from build123d import *

# Parameters (mm, degrees)
SKETCH1_W           = 100
SKETCH1_H           = 60
BOSS_EXTRUDE1_DEPTH = 5
CUT_EXTRUDE2_START  = 5
SKETCH2_R           = 4
CUT_EXTRUDE2_DEPTH  = 64.523499554
CUT_EXTRUDE4_START  = 5
SKETCH3_R           = 10
CUT_EXTRUDE4_DEPTH  = 64.523499554
CHAMFER1_SIZE       = 1


with BuildPart() as part:
    # Sketch1 → Boss-Extrude1 (new, symmetric)
    with BuildSketch(Plane(origin=(0, 0, 0), x_dir=(0, 1, 0), z_dir=(0, 0, 1))):
        Rectangle(SKETCH1_W, SKETCH1_H)
    extrude(amount=BOSS_EXTRUDE1_DEPTH, both=True)

    # Sketch2 → Cut-Extrude2 (cut, through all)
    with BuildSketch(Plane(origin=(0, 0, 0), x_dir=(0, 1, 0), z_dir=(0, 0, 1)).offset(CUT_EXTRUDE2_START)):
        with Locations(Location((-40, -20, 0), (0, 0, 270))):
            Circle(SKETCH2_R)
        with Locations(Location((40, -20, 0), (0, 0, 270))):
            Circle(SKETCH2_R)
        with Locations(Location((-40, 20, 0), (0, 0, 270))):
            Circle(SKETCH2_R)
        with Locations(Location((40, 20, 0), (0, 0, 270))):
            Circle(SKETCH2_R)
    extrude(amount=-CUT_EXTRUDE2_DEPTH, mode=Mode.SUBTRACT)

    # Sketch3 → Cut-Extrude4 (cut, through all)
    with BuildSketch(Plane(origin=(0, 0, 0), x_dir=(0, 1, 0), z_dir=(0, 0, 1)).offset(CUT_EXTRUDE4_START)):
        with Locations(Location((0, 0, 0), (0, 0, 270))):
            Circle(SKETCH3_R)
    extrude(amount=-CUT_EXTRUDE4_DEPTH, mode=Mode.SUBTRACT)

    # Chamfer1
    chamfer1_edges = [part.edges().sort_by_distance(p)[0] for p in [
        (-10, 0, -5),
        (-10, 0, 5),
    ]]
    chamfer(chamfer1_edges, length=CHAMFER1_SIZE)


solid = part.part
Could you check a few things on this model? Use its own coordinates, in mm. Round coordinates to 2 decimals unless told otherwise and drop trailing zeros. Write each loop counter-clockwise with the first axis right and the second up, starting at its lowest first coordinate (ties: lowest second). Pieces come first, ordered by that corner, then holes. Notation, with made-up numbers: (-24.75, 18) - (28.25, 18) arc R19 ccw to (28.25, 50) - close; hole circle Ø7 at (-40, 60.25). An arc over 180 degrees is marked (long way). Put each result on its own line as item: value. Start each with the question number.
(1) Will this pin go through, and if not, where does the flat tip stop? pin 1 (6.5 mm diameter, centred on x = 20, y = -40, fed in from +Z).
(2) I want a section at C-C, the plane y = 0. Please give me the cut outline in (x, z), plus the area to 3 significant figures.
(3) Thinking about a two-plate mould opening in X: for faces 1 (the flat face through (30, -1, 0)), 2 (the flat face through (0, -50, 0)), 3 (the cylindrical face through (-20.521, 43.966, 0.07)), which applies, released by +X, released by -X, zero draft, split by the parting line, or undercut?
(4) I need wall thicknesses on probe 1 along Y at (x, z) = (-20, -2.5); probe 2 along Y at (x, z) = (-23, -3.75); probe 3 along Y at (x, z) = (-3.5, 3.5). Which ranges of each line are inside material? Lowest first, please.
(5) I want a section at D-D, the plane x = 0. Please give me the cut outline in (y, z), plus the area to 3 significant figures.
(6) I want a section at A-A, the plane y = -40. Please give me the cut outline in (x, z).
(7) I want a section at B-B, the plane x = 20. Please give me the cut outline in (y, z).
Here are the results:
1. pin 1: passes through
2. outline: (-30, -5) - (-11, -5) - (-10, -4) - (-10, 4) - (-11, 5) - (-30, 5) - close; (10, -4) - (11, -5) - (30, -5) - (30, 5) - (11, 5) - (10, 4) - close
2. area: 398 mm^2
3. face 1: released by +X
3. face 2: zero draft
3. face 3: undercut
4. probe 1: y = -50 to -44, -36 to 36, 44 to 50
4. probe 2: y = -50 to -42.65, -37.35 to 37.35, 42.65 to 50
4. probe 3: y = -50 to -9.37, 9.37 to 50
5. outline: (-50, -5) - (-11, -5) - (-10, -4) - (-10, 4) - (-11, 5) - (-50, 5) - close; (10, -4) - (11, -5) - (50, -5) - (50, 5) - (11, 5) - (10, 4) - close
5. area: 798 mm^2
6. outline: (-30, -5) - (-24, -5) - (-24, 5) - (-30, 5) - close; (-16, -5) - (16, -5) - (16, 5) - (-16, 5) - close; (24, -5) - (30, -5) - (30, 5) - (24, 5) - close
7. outline: (-50, -5) - (-44, -5) - (-44, 5) - (-50, 5) - close; (-36, -5) - (36, -5) - (36, 5) - (-36, 5) - close; (44, -5) - (50, -5) - (50, 5) - (44, 5) - close
